Autodesk Inventor part; units mm, degrees
ref_plane "YZ Plane" through (0, 0, 0) normal (1, 0, 0) x (0, 1, 0)
ref_plane "XZ Plane" through (0, 0, 0) normal (0, 1, 0) x (-1, 0, 0)
ref_plane "XY Plane" through (0, 0, 0) normal (0, 0, 1) x (1, 0, 0)
sketch "Sketch1" plane through (0, 0, 0) normal (0, 0, 1) x (1, 0, 0)
  line L0 (0, 0) -> (11.7, 0)
  arc A0 (11.7, 0) -> (13.5, 1.8) centre (11.7, 1.8) ccw
  line L1 (13.5, 1.8) -> (13.5, 5.7)
  arc A1 (14.3, 6.5) -> (13.5, 5.7) centre (14.3, 5.7) ccw
  line L2 (14.3, 6.5) -> (17.5, 6.5)
  line L3 (17.5, 6.5) -> (17.5, 7.5)
  line L4 (17.5, 7.5) -> (14.3, 7.5)
  arc A2 (14.3, 7.5) -> (12.5, 5.7) centre (14.3, 5.7) ccw
  line L5 (12.5, 5.7) -> (12.5, 1.8)
  arc A3 (11.7, 1) -> (12.5, 1.8) centre (11.7, 1.8) ccw
  line L6 (11.7, 1) -> (0, 1)
  line L7 (0, 1) -> (0, 0)
  dimension "d0" = 1
  dimension "d2" = 0.8
  dimension "d3" = 25
  dimension "d4" = 35
  dimension "d5" = 7.5
extrude "Extrusion1" add sketch "Sketch1" along normal blind 10
mirror "Mirror1" about plane through (0, 1, 0) normal (-1, 0, 0) of "Extrusion1"
properties part number "din_rail"
Design review of the part built by this model. Coordinates are the model's own, in mm. A direction names the side the tool comes from. Coordinates: 2 decimals unless noted, no trailing zeros. Write each loop counter-clockwise with the first axis right and the second up, starting at its lowest first coordinate (ties: lowest second). Pieces come first, ordered by that corner, then holes.
1) Add section C-C (x = 9.5). Write out the cut boundary in (y, z).
2) Add section A-A (y = 3). Write out the cut boundary in (x, z), plus the area to 3 significant figures.
3) Add section B-B (z = 3.25). Write out the cut boundary in (x, y).
4) To check wall thickness, follow L1, parallel to X at y = 3.75, z = 0.5; L2, parallel to Y at x = 7, z = 6.25; L3, parallel to X at y = 6, z = 7. State the ranges of each line that lie inside material, in increasing order.
5) Insertion check: pin 1 (5 mm diameter, centred on x = 1.5, z = 7, fed in from +Y); pin 2 (1 mm diameter, centred on x = 15.5, z = 7, fed in from -Y); pin 3 (1.2 mm diameter, centred on y = 4.5, z = 3, fed in from +X). Each pin has a flat end and moves straight along its axis. Give the tip position at first contact, or say it passes through.
6) Machinability: for faces 1 (the flat face through (12.5, 4, 5)), 2 (the flat face through (-16, 7.5, 5)), 3 (the flat face through (-16, 6.5, 5)), which of the approach directions +Z, -Z, +X, -X, +Y, -Y give a long, thin tool a straight path to every point of the face, cutting with its end or side? Answer none if there is none.
7) Mouldability with a two-part tool opening along X and no side actions: class faces 4 (the flat face through (13.5, 4, 5)), 5 (the flat face through (-0.1, 0.4, 10)), 6 (the cylindrical face through (-13.041, 6.987, 4.93)) as +X half, -X half, draft (parallel to the pull), parting line (faces both ways), or undercut.
8) Add section D-D (x = 14). Write out the cut boundary in (y, z), plus the area to 3 significant figures.
Check result:
1. outline: (0, 0) - (1, 0) - (1, 10) - (0, 10) - close
2. outline: (-13.5, 0) - (-12.5, 0) - (-12.5, 10) - (-13.5, 10) - close; (12.5, 0) - (13.5, 0) - (13.5, 10) - (12.5, 10) - close
2. area: 20.0 mm2
3. outline: (-17.5, 6.5) - (-14.3, 6.5) arc R0.8 cw to (-13.5, 5.7) - (-13.5, 1.8) arc R1.8 ccw to (-11.7, 0) - (11.7, 0) arc R1.8 ccw to (13.5, 1.8) - (13.5, 5.7) arc R0.8 cw to (14.3, 6.5) - (17.5, 6.5) - (17.5, 7.5) - (14.3, 7.5) arc R1.8 ccw to (12.5, 5.7) - (12.5, 1.8) arc R0.8 cw to (11.7, 1) - (-11.7, 1) arc R0.8 cw to (-12.5, 1.8) - (-12.5, 5.7) arc R1.8 ccw to (-14.3, 7.5) - (-17.5, 7.5) - close
4. L1: x = -13.5 to -12.5, 12.5 to 13.5
4. L2: y = 0 to 1
4. L3: x = -13.56 to -12.53, 12.53 to 13.56
5. pin 1: stops at y = 1
5. pin 2: stops at y = 6.5
5. pin 3: stops at x = 13.5
6. face 1: +Z, -Z, +Y
6. face 2: +Z, -Z, +X, -X, +Y
6. face 3: +Z, -Z, -X, -Y
7. face 4: +X half
7. face 5: draft
7. face 6: undercut
8. outline: (6.44, 0) - (7.47, 0) - (7.47, 10) - (6.44, 10) - close
8. area: 10.3 mm2
